Design review of the part built by this model. Coordinates are the model's own, in mm. Face numbers are marked on the shaded views. A direction names the side the tool comes from. Give positions to 0.01 mm unless a question says otherwise; leave off trailing zeros. Write each loop counter-clockwise with the first axis right and the second up, starting at its lowest first coordinate (ties: lowest second). Pieces come first, ordered by that corner, then holes. Notation, with made-up numbers: M 23.5,-36.5 L 58.5,-36.5 A13 cw 58.5,-23.5 Z; hole C 54,74.25 d3. An arc over 180 degrees is marked long. Answer in a Markdown table with one row per item.
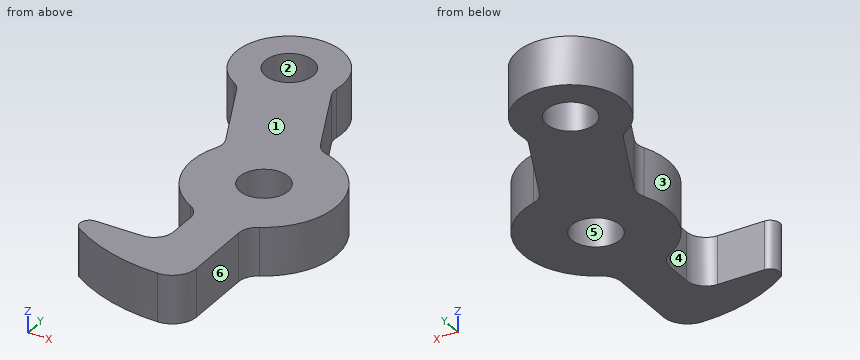
```python
from build123d import *

# Parameters (mm, degrees)
SKETCH1_R           = 3.175
BOSS_EXTRUDE1_DEPTH = 3.175
FILLET1_R           = 2.54
FILLET2_R           = 1.27


with BuildPart() as part:
    # Sketch1 → Boss-Extrude1 (new, symmetric)
    with BuildSketch(Plane.XY):
        with BuildLine():
            Line((1.499199331, 9.406275903), (-3.9943168, 21.187159265))
            ThreePointArc((-3.9943168, 21.187159265), (-13.686492406, 29.350777683), (-13.662808272, 16.678667649))
            Line((-13.662808272, 16.678667649), (-8.169292141, 4.897784287))
            ThreePointArc((-8.169292141, 4.897784287), (-8.962323495, -3.225272479), (-3.175, -8.980256121))
            Line((-3.175, -8.980256121), (-3.175, -16.773611102))
            Line((-3.175, -16.773611102), (-15.531438137, -16.773611102))
            ThreePointArc((-15.531438137, -16.773611102), (-8.340708909, -21.284082665), (0, -22.86))
            ThreePointArc((0, -22.86), (2.24506403, -21.93006403), (3.175, -19.685))
            Line((3.175, -19.685), (3.175, -8.980256121))
            ThreePointArc((3.175, -8.980256121), (9.485682623, 0.864552013), (1.499199331, 9.406275903))
        make_face()
        with Locations((-10.734503848, 23.020217791)):
            Circle(SKETCH1_R, mode=Mode.SUBTRACT)
        Circle(SKETCH1_R, mode=Mode.SUBTRACT)
    extrude(amount=BOSS_EXTRUDE1_DEPTH, both=True)

    # Fillet1
    fillet1_edges = [part.edges().sort_by_distance(p)[0] for p in [
        (-3.175, -16.773611102, 0),
        (-3.175, -8.980256121, 0),
        (-8.169292141, 4.897784287, 0),
        (-13.662808272, 16.678667649, 0),
        (-3.9943168, 21.187159265, 0),
        (1.499199331, 9.406275903, 0),
        (3.175, -8.980256121, 0),
    ]]
    fillet(fillet1_edges, radius=FILLET1_R)

    # Fillet2
    fillet2_edges = [part.edges().sort_by_distance(p)[0] for p in [
        (-15.531438137, -16.773611102, 0),
    ]]
    fillet(fillet2_edges, radius=FILLET2_R)


solid = part.part
```
1) Add section A-A (y = 25). Write out the cut boundary in (x, z) (3 decimals).
Geometry says:
| item | result |
|---|---|
| outline | M -17.433,-3.175 L -13.217,-3.175 L -13.217,3.175 L -17.433,3.175 Z; M -8.252,-3.175 L -4.036,-3.175 L -4.036,3.175 L -8.252,3.175 Z |
2) For the marked faces 4, 5 and 6, list the 3-axis set-ups (+Z, -Z, +X, -X, +Y, -Y) from which the entire face can be reached by the end or side of a thin tool; tool diameter is ignored.
Geometry says:
| item | result |
|---|---|
| face 4 | +Z, -Z, -X |
| face 5 | +Z, -Z |
| face 6 | +Z, -Z, +X, -Y |
3) Insertion check: P1, Ø1, axis at y = 15, z = 0.5, coming from the +X side; P2, Ø1.8, axis at y = -12, z = 0.5, coming from the -X side (3 decimals); P3, Ø1, axis at x = -7.5, z = -0.5, coming from the -Y side. Each pin has a flat end and moves straight along its axis. Give the tip position at first contact, or say it passes through.
Geometry says:
| item | result |
|---|---|
| P1 | x = -0.88 |
| P2 | x = -3.175 |
| P3 | y = -21.76 |
4) Add section D-D (y = 16.5). Write out the cut boundary in (x, z) (3 decimals).
Geometry says:
| item | result |
|---|---|
| outline | M -13.687,-3.175 L -1.809,-3.175 L -1.809,3.175 L -13.687,3.175 Z |
5) To check wall thickness, follow probe 1 along X at (y, z) = (-13.5, 1) (3 decimals); probe 2 along Y at (x, z) = (2.5, 1.25); probe 3 along Y at (x, z) = (0, 1) (3 decimals). State the ranges of each line that lie inside material, in increasing order. Write a range as [from, to].
Geometry says:
| item | result |
|---|---|
| probe 1 | [-3.175, 3.175] |
| probe 2 | [-21.64, -1.96], [1.96, 9.19] |
| probe 3 | [-22.86, -3.175], [3.175, 12.621] |
6) The part is to be moulded in two halves that separate along X. For the marked faces 1, 2 and 3, say which applies: released by +X, released by -X, zero draft, split by the parting line, or undercut.
Geometry says:
| item | result |
|---|---|
| face 1 | zero draft |
| face 2 | undercut |
| face 3 | released by -X |
7) Add section C-C (z = -1.5). Count the separate pieces of the cut face and the enclosed holes in it, and give its area (3 significant figures).
Geometry says:
| item | result |
|---|---|
| separate pieces | 1 |
| enclosed holes | 2 |
| area | 613 mm^2 |
8) Add section B-B (x = -2.5). Write out the cut boundary in (y, z) (3 decimals).
Geometry says:
| item | result |
|---|---|
| outline | M -22.723,-3.175 L -1.957,-3.175 L -1.957,3.175 L -22.723,3.175 Z; M 1.957,-3.175 L 17.983,-3.175 L 17.983,3.175 L 1.957,3.175 Z |
